Autodesk Inventor part; units mm, degrees
ref_plane "Work Plane1" through (16.25, 0, 0) normal (1, 0, 0) x (0, 1, 0)
ref_plane "XZ Plane" through (0, 0, 0) normal (0, 1, 0) x (-1, 0, 0)
ref_plane "XY Plane" through (0, 0, 0) normal (0, 0, 1) x (1, 0, 0)
sketch "Sketch1" plane through (0, 0, 0) normal (0, 1, 0) x (-1, 0, 0)
  circle A0 centre (0, 0) radius 16
  circle A1 centre (0, 0) radius 12.5
  dimension "d0" = 32
  dimension "d1" = 25
extrude "Extrusion1" add sketch "Sketch1" along normal blind 3
ref_plane "Work Plane1" through (16.25, 0, 0) normal (1, 0, 0) x (0, 1, 0)
sketch "Sketch2" plane through (16.25, 0, 0) normal (1, 0, 0) x (0, 1, 0)
  line L0 (0, 0) -> (3, 5.1962)
  line L1 (3, -16) -> (3, 16)
  line L2 (0, -12.5) -> (0, 12.5)
  line L3 (0, 0) -> (0, -4)
  line L4 (0, 16) -> (0, -16)
  line L5 (0, -4) -> (3, 1.1962)
  line L6 (3, 5.1962) -> (3, 1.1962)
  dimension "d10" = 2
  dimension "d11" = 30
extrude "Extrusion2" cut sketch "Sketch2" against normal blind 9
properties part number "PistonRing" material "Stainless Steel"
Work out the finished part from the listing and answer in its coordinate system (mm). Give positions to 0.01 mm unless a question says otherwise; leave off trailing zeros. Loops run counter-clockwise (first coordinate to the right, second up) from the corner with the lowest first, then second, coordinate; pieces in that order, holes last. Notation, with made-up numbers: (-18.5, 58.5) - (26.5, 58.5) arc R24 ccw to (26.5, 83.5) - close; hole circle Ø4 at (32, 85). An arc over 180 degrees is marked (long way). Answer in a Markdown table with one row per item.
(1) Consider L1, parallel to Z at x = -6.5, y = 0.55; L2, parallel to Z at x = -4, y = 2.4; L3, parallel to X at y = 1.5, z = -11.5. Determine where each line is inside the solid, lowest interval first. Write a range as [from, to].
Results list:
| item | result |
|---|---|
| L1 | z = [-14.62, -10.68], [10.68, 14.62] |
| L2 | z = [-15.49, -11.84], [11.84, 15.49] |
| L3 | x = [-11.12, -4.9], [4.9, 11.12] |
(2) Section A-A (x = 0) is taken. Give the vertices of the cut face in (y, z).
Results list:
| item | result |
|---|---|
| outline | (0, -16) - (3, -16) - (3, -12.5) - (0, -12.5) - close; (0, 12.5) - (3, 12.5) - (3, 16) - (0, 16) - close |
(3) Section C-C (y = 2.5) is taken. Give the vertices of the cut face in (x, z), and give its area (3 significant figures).
Results list:
| item | result |
|---|---|
| outline | (11.73, 4.33) - (15.4, 4.33) arc R16 ccw (long way) to (16, 0.33) - (12.5, 0.33) arc R12.5 cw (long way) to start |
| area | 299 mm² |
(4) For a pull along Y with two mould halves and no side action, classify faces 1 (the face through (-12, 3, 5)), 2 (the face through (-8, 0, 10)), 3 (the face through (13.7, 1.5, 2.6)) as pulls with the +Y half, pulls with the -Y half, needs draft (parallel to the pull), parting line crosses it, or undercut.
Results list:
| item | result |
|---|---|
| face 1 | pulls with the +Y half |
| face 2 | pulls with the -Y half |
| face 3 | undercut |
(5) Section B-B (z = -12) is taken. Give the vertices of the cut face in (x, y), and give its area (3 significant figures).
Results list:
| item | result |
|---|---|
| outline | (-10.58, 0) - (-3.5, 0) - (-3.5, 3) - (-10.58, 3) - close; (3.5, 0) - (10.58, 0) - (10.58, 3) - (3.5, 3) - close |
| area | 42.5 mm² |
(6) Flat-ended cylindrical pins translate along their axes: pin 1 Ø12 at (x, z) = (2, 8) entering from -Y; pin 2 Ø1 at (y, z) = (0.5, -7) entering from +X; pin 3 Ø8 at (x, z) = (-0.5, 7.5) entering from -Y. Find the tip coordinate at first contact, or state that the pin passes through.
Results list:
| item | result |
|---|---|
| pin 1 | stops at y = 0 |
| pin 2 | stops at x = 14.62 |
| pin 3 | passes through |
